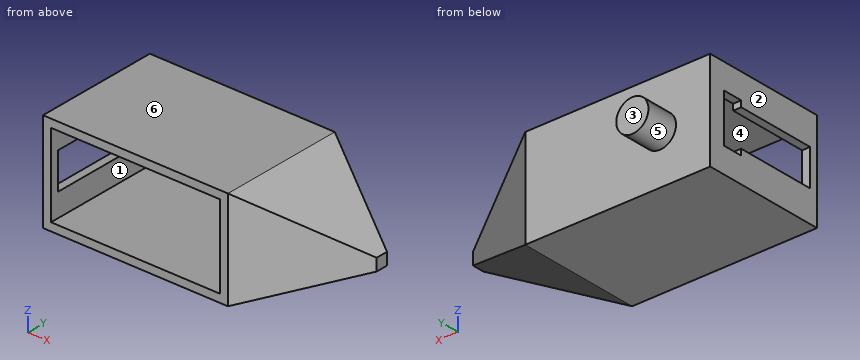
from build123d import *

# Parameters (mm, degrees)
SKETCH1_W           = 46
SKETCH1_H           = 24.5
BODY_DEPTH          = 31
SKETCH3_W           = 42
SKETCH3_H           = 20.5
SERVO_HOLE_DEPTH    = 29
CUT_EXTRUDE3_DEPTH  = 29
SKETCH6_R           = 4
BOSS_EXTRUDE3_DEPTH = 8


with BuildPart() as part:
    # Sketch1 → Body (new body)
    with BuildSketch(Plane(origin=(0, 0, 0), x_dir=(1, 0, 0), z_dir=(0, 1, 0))):
        Rectangle(SKETCH1_W, SKETCH1_H)
    extrude(amount=BODY_DEPTH)

    # Sketch3 → Servo Hole (cut)
    with BuildSketch(Plane(origin=(0, 0, 0), x_dir=(1, 0, 0), z_dir=(0, 1, 0))):
        Rectangle(SKETCH3_W, SKETCH3_H)
    extrude(amount=SERVO_HOLE_DEPTH, mode=Mode.SUBTRACT)

    # Point → section 0 of loft1
    with BuildSketch(Plane(origin=(48, 0, 0), x_dir=(0, 0, -1), z_dir=(1, 0, 0)), mode=Mode.PRIVATE) as loft1_s0:
        with BuildLine():
            Line((-1.5, 14), (1.5, 14))
            Line((1.5, 14), (1.5, 17))
            Line((1.5, 17), (-1.5, 17))
            Line((-1.5, 17), (-1.5, 14))
        make_face()
    # loft up to a face of the part (loft1)
    loft([loft1_s0.sketch, part.faces().sort_by_distance((23, 15.5, 0))[0]])

    # Sketch5 → Cut-Extrude3 (cut)
    with BuildSketch(Plane.ZY.offset(23)):
        Polygon((-6, 27), (6, 27), (6, 22), (4.5, 22), (4.5, 2), (-4.5, 2), (-4.5, 22), (-6, 22), align=None)
    extrude(amount=-CUT_EXTRUDE3_DEPTH, mode=Mode.SUBTRACT)

    # Sketch6 → Boss-Extrude3 (add)
    with BuildSketch(Plane(origin=(0, 31, 0), x_dir=(1, 0, 0), z_dir=(0, 1, 0))):
        with Locations(Location((-10.5, 0, 0), (0, 0, 90))):
            Circle(SKETCH6_R)
    extrude(amount=BOSS_EXTRUDE3_DEPTH)


solid = part.part
Input: part model. Units: mm. Frame: model coordinates. Face numbers are marked on the shaded views. A direction names the side the tool comes from. Give positions to 0.01 mm unless a question says otherwise; leave off trailing zeros. Order: outer loops, then holes, each group sorted by start corner. A loop starts at its lowest first (then second) coordinate and runs counter-clockwise, first axis right, second up. Notation, with made-up numbers: M -5,38 L 23,38 A34 cw 23,76 Z; hole C -31,-7 d5. An arc over 180 degrees is marked long. Answer as a JSON object with one key per item and string values.
1. Ray query, line 1 (Z direction, x = -14, y = 14); line 2 (Y direction, x = 7.5, z = -2.5); line 3 (X direction, y = 16, z = -8.25). Return the intervals inside material, ascending. Write a range as [from, to].
Result sheet:
{"line 1": "[-12.25, -10.25], [10.25, 12.25]", "line 2": "[29, 31]", "line 3": "[-23, -21], [21, 32.3]"}
2. Cut plane A-A, the plane x = -10.5. Output: boundary loops of the cut face in (y, z).
Result sheet:
{"outline": "M 0,-12.25 L 31,-12.25 L 31,-4 L 39,-4 L 39,4 L 31,4 L 31,12.25 L 0,12.25 L 0,10.25 L 29,10.25 L 29,-10.25 L 0,-10.25 Z"}
3. Pull-direction query (X, two-part tool) for the marked faces 1, 2 and 3; classes: +X half, -X half, draft (parallel to the pull), parting line (faces both ways), or undercut.
Result sheet:
{"face 1": "undercut", "face 2": "-X half", "face 3": "draft"}
4. Cut plane B-B, the plane y = 33. Output: boundary loops of the cut face in (x, z), and give its area (3 significant figures).
Result sheet:
{"outline": "C -10.5,0 d8", "area": "50.3 mm²"}
5. Reachability of the marked faces 4, 5 and 6 from +Z, -Z, +X, -X, +Y, -Y: full face, straight path, thin tool, end or side. Return the list, or none.
Result sheet:
{"face 4": "-Y", "face 5": "+Y", "face 6": "+Z, +X, -X, +Y, -Y"}
6. Cut plane C-C, the plane x = 9. Output: boundary loops of the cut face in (y, z).
Result sheet:
{"outline": "M 0,-12.25 L 31,-12.25 L 31,12.25 L 0,12.25 L 0,10.25 L 29,10.25 L 29,-10.25 L 0,-10.25 Z"}
7. First-contact query: P1, Ø2, axis at x = 14.5, z = 3.5, coming from the -Y side; P2, Ø3, axis at x = 17.5, z = 8.5, coming from the +Y side; P3, Ø1, axis at y = 10, z = -9.5, coming from the +X side. Flat tips, straight axial feed; report the tip coordinate or a pass-through.
Result sheet:
{"P1": "y = 29", "P2": "y = 31", "P3": "x = 30.56"}
